```python
from build123d import *

# Parameters (mm, degrees)
ESQUISSE2_R        = 9.525
ESQUISSE2_R_2      = 4.8514
BOSS_EXTRU_1_DEPTH = 12.7
CONG_2_R           = 0.5


with BuildPart() as part:
    # Esquisse2 → Boss.-Extru.1 (new body, symmetric)
    with BuildSketch(Plane(origin=(0, 0, 0), x_dir=(1, 0, 0), z_dir=(0, 1, 0))):
        Circle(ESQUISSE2_R)
        Circle(ESQUISSE2_R_2, mode=Mode.SUBTRACT)
    extrude(amount=BOSS_EXTRU_1_DEPTH, both=True)

    # Congé2
    cong_2_edges = [part.edges().sort_by_distance(p)[0] for p in [
        (-9.525, -12.7, 0),
        (-9.525, 12.7, 0),
        (-4.8514, -12.7, 0),
        (-4.8514, 12.7, 0),
    ]]
    fillet(cong_2_edges, radius=CONG_2_R)


solid = part.part
```
Verification items for the finished model (mm, model axes). Round coordinates to 2 decimals unless told otherwise and drop trailing zeros. Write each loop counter-clockwise with the first axis right and the second up, starting at its lowest first coordinate (ties: lowest second). Pieces come first, ordered by that corner, then holes. Notation, with made-up numbers: (-24, 89.5) -> (3, 89.5) arc R15 ccw to (3, 105.5) -> close; hole circle Ø4 at (9.25, 71.25). An arc over 180 degrees is marked (long way). Write each question's results on one line, items separated by ' | '. Start each with the question number.
1. Draft check along X on faces 1 (the flat face through (4, 12.7, 4)), 2 (the cylindrical face through (4.627, -0.171, -1.457)), 3 (the cylindrical face through (-7.559, 0.171, 5.796)). Enter one of: +X half, -X half, draft (parallel to the pull), parting line (faces both ways), or undercut.
2. Material ranges on probe 1 along Z at (x, y) = (0, 1.25) (3 decimals); probe 2 along X at (y, z) = (-8.25, -2.5), recorded low to high. Write a range as from..to.
3. Cross-section at A-A (z = 0). Enter the section's corners in (x, y) (3 decimals).
4. Cross-section at B-B (x = 0). Enter the section's corners in (y, z) (3 decimals), then the cut area to 3 significant figures.
5. Cross-section at C-C (y = -9). Enter the section's corners in (x, z) (3 decimals).
6. Depth check by flat-ended pin: P1, Ø1, axis at y = -2, z = -1, coming from the +X side; P2, Ø3, axis at x = 7, y = 6.5, coming from the +Z side; P3, Ø1.5, axis at y = -6, z = 7.5, coming from the -X side; P4, Ø8, axis at x = 0, z = 0, coming from the -Y side. Enter the tip coordinate at first touch or a pass-through.
Solutions:
1) face 1: draft | face 2: undercut | face 3: parting line
2) probe 1: z = -9.525..-4.851, 4.851..9.525 | probe 2: x = -9.19..-4.16, 4.16..9.19
3) outline: (-9.525, -12.2) arc R0.5 ccw to (-9.025, -12.7) -> (-5.351, -12.7) arc R0.5 ccw to (-4.851, -12.2) -> (-4.851, 12.2) arc R0.5 ccw to (-5.351, 12.7) -> (-9.025, 12.7) arc R0.5 ccw to (-9.525, 12.2) -> close; (4.851, -12.2) arc R0.5 ccw to (5.351, -12.7) -> (9.025, -12.7) arc R0.5 ccw to (9.525, -12.2) -> (9.525, 12.2) arc R0.5 ccw to (9.025, 12.7) -> (5.351, 12.7) arc R0.5 ccw to (4.851, 12.2) -> close
4) outline: (-12.7, -9.025) arc R0.5 ccw to (-12.2, -9.525) -> (12.2, -9.525) arc R0.5 ccw to (12.7, -9.025) -> (12.7, -5.351) arc R0.5 ccw to (12.2, -4.851) -> (-12.2, -4.851) arc R0.5 ccw to (-12.7, -5.351) -> close; (-12.7, 5.351) arc R0.5 ccw to (-12.2, 4.851) -> (12.2, 4.851) arc R0.5 ccw to (12.7, 5.351) -> (12.7, 9.025) arc R0.5 ccw to (12.2, 9.525) -> (-12.2, 9.525) arc R0.5 ccw to (-12.7, 9.025) -> close | area: 237 mm2
5) outline: circle Ø19.05 at (0, 0); hole circle Ø9.703 at (0, 0)
6) P1: stops at x = 9.51 | P2: stops at z = 7.78 | P3: stops at x = -6.72 | P4: passes through
